from build123d import *

# Parameters (mm, degrees)
SKETCH1_W           = 150
SKETCH1_H           = 100
BOSS_EXTRUDE1_DEPTH = 3
SKETCH2_W           = 20
SKETCH2_H           = 3
CUT_EXTRUDE1_DEPTH  = 3
SKETCH3_W           = 3
SKETCH3_H           = 17
CUT_EXTRUDE2_DEPTH  = 3
SKETCH5_R           = 4.5
CUT_EXTRUDE4_DEPTH  = 30.5
SKETCH6_R           = 4.5
CUT_EXTRUDE5_DEPTH  = 10
SKETCH7_R           = 1
CUT_EXTRUDE6_DEPTH  = 10
SKETCH9_W           = 29.951530893
SKETCH9_H           = 14.675464834
CUT_EXTRUDE7_DEPTH  = 10
SKETCH10_W          = 6.632124697
SKETCH10_H          = 15.189704953
CUT_EXTRUDE8_DEPTH  = 10
CAVITY1_START       = -15
CAVITY1_OUTLINE_W   = 15
CAVITY1_OUTLINE_H   = 3
CAVITY1_DEPTH       = 3
CAVITY1_START_2     = 12
CAVITY1_2_OUTLINE_W = 15
CAVITY1_2_OUTLINE_H = 3
CAVITY1_2_DEPTH     = 3
SKETCH11_W          = 8.771519761
SKETCH11_H          = 15.403644459
CUT_EXTRUDE9_DEPTH  = 10


# Read off the part's stored shape, not the designer's step: Cavity1
with BuildPart() as part:
    # Sketch1 → Boss-Extrude1 (new body)
    with BuildSketch(Plane.XY):
        Rectangle(SKETCH1_W, SKETCH1_H)
    extrude(amount=BOSS_EXTRUDE1_DEPTH)

    # Sketch2 → Cut-Extrude1 (cut)
    with BuildSketch(Plane.XY.offset(3)):
        with Locations((65, 48.5)):
            Rectangle(SKETCH2_W, SKETCH2_H)
        with Locations((-65, 48.5)):
            Rectangle(SKETCH2_W, SKETCH2_H)
        with Locations((-65, -48.5)):
            Rectangle(SKETCH2_W, SKETCH2_H)
        with Locations((65, -48.5)):
            Rectangle(SKETCH2_W, SKETCH2_H)
    extrude(amount=-CUT_EXTRUDE1_DEPTH, mode=Mode.SUBTRACT)

    # Sketch3 → Cut-Extrude2 (cut)
    with BuildSketch(Plane.XY.offset(3)):
        with Locations((-73.5, 38.5)):
            Rectangle(SKETCH3_W, SKETCH3_H)
        with Locations((-73.5, -38.5)):
            Rectangle(SKETCH3_W, SKETCH3_H)
        with Locations((73.5, 38.5)):
            Rectangle(SKETCH3_W, SKETCH3_H)
        with Locations((73.5, -38.5)):
            Rectangle(SKETCH3_W, SKETCH3_H)
    extrude(amount=-CUT_EXTRUDE2_DEPTH, mode=Mode.SUBTRACT)

    # Sketch5 → Cut-Extrude4 (cut)
    with BuildSketch(Plane.XY.offset(3)):
        with Locations((50, 17.807715926)):
            Circle(SKETCH5_R)
        with Locations((-50, 17.807715926)):
            Circle(SKETCH5_R)
    extrude(amount=-CUT_EXTRUDE4_DEPTH, mode=Mode.SUBTRACT)

    # Sketch6 → Cut-Extrude5 (cut)
    with BuildSketch(Plane(origin=(0, 0, 0), x_dir=(-1, 0, 0), z_dir=(0, 0, -1))):
        with Locations((26.644067797, -29.026784983)):
            Circle(SKETCH6_R)
        with Locations((-26.644067797, -29.026784983)):
            Circle(SKETCH6_R)
    extrude(amount=-CUT_EXTRUDE5_DEPTH, mode=Mode.SUBTRACT)

    # Sketch7 → Cut-Extrude6 (cut)
    with BuildSketch(Plane.XY.offset(3)):
        with Locations((0, 18.473215017)):
            Circle(SKETCH7_R)
        with Locations((0, -29.026784983)):
            Circle(SKETCH7_R)
    extrude(amount=-CUT_EXTRUDE6_DEPTH, mode=Mode.SUBTRACT)

    # Sketch9 → Cut-Extrude7 (cut)
    with BuildSketch(Plane.XY.offset(3)):
        with Locations((52.201239556, -7.337732417)):
            Rectangle(SKETCH9_W, SKETCH9_H)
    extrude(amount=-CUT_EXTRUDE7_DEPTH, mode=Mode.SUBTRACT)

    # Sketch10 → Cut-Extrude8 (cut)
    with BuildSketch(Plane.XY.offset(3)):
        with Locations((0.32090926, -24.837591387)):
            Rectangle(SKETCH10_W, SKETCH10_H)
    extrude(amount=-CUT_EXTRUDE8_DEPTH, mode=Mode.SUBTRACT)

    # Cavity1 outline → Cavity1 (cut)
    with BuildSketch(Plane.YZ.offset(CAVITY1_START)):
        with Locations((-24.318956618, 1.5)):
            Rectangle(CAVITY1_OUTLINE_W, CAVITY1_OUTLINE_H)
    extrude(amount=CAVITY1_DEPTH, mode=Mode.SUBTRACT)

    # Cavity1 2 outline → Cavity1 2 (cut)
    with BuildSketch(Plane.YZ.offset(CAVITY1_START_2)):
        with Locations((-24.318956618, 1.5)):
            Rectangle(CAVITY1_2_OUTLINE_W, CAVITY1_2_OUTLINE_H)
    extrude(amount=CAVITY1_2_DEPTH, mode=Mode.SUBTRACT)

    # Sketch11 → Cut-Extrude9 (cut)
    with BuildSketch(Plane.XY.offset(3)):
        with Locations((0.32090926, 13.778489515)):
            Rectangle(SKETCH11_W, SKETCH11_H)
    extrude(amount=-CUT_EXTRUDE9_DEPTH, mode=Mode.SUBTRACT)


solid = part.part
Can you work these out from the model? Positions are in its coordinate system, mm. A direction names the side the tool comes from. Give positions to 0.01 mm unless a question says otherwise; leave off trailing zeros. Loops run counter-clockwise (first coordinate to the right, second up) from the corner with the lowest first, then second, coordinate; pieces in that order, holes last. Notation, with made-up numbers: (69, 79) - (92, 79) arc R15 ccw to (92, 104) - close; hole circle Ø8 at (59, 49.25). An arc over 180 degrees is marked (long way). Answer as a JSON object with one key per item and string values.
Q1. If we mould it in two halves opening along Y, with no side actions, what happens to faces 1 (the flat face through (52, 0, 2)), 2 (the flat face through (-1, 1, 3)), 3 (the flat face through (-74, -30, 2))? For each: pulls with the +Y half, pulls with the -Y half, needs draft (parallel to the pull), parting line crosses it, or undercut.
Geometry says:
{"face 1": "undercut", "face 2": "needs draft", "face 3": "pulls with the -Y half"}
Q2. Imagine slicing it at D-D on x = 50. Write out the boundary of the cut face in (y, z).
Geometry says:
{"outline": "(-50, 0) - (-14.68, 0) - (-14.68, 3) - (-50, 3) - close; (0, 0) - (13.31, 0) - (13.31, 3) - (0, 3) - close; (22.31, 0) - (50, 0) - (50, 3) - (22.31, 3) - close"}
Q3. Imagine slicing it at B-B on y = -22. Write out the boundary of the cut face in (x, z), plus the area to 3 significant figures.
Geometry says:
{"outline": "(-75, 0) - (-15, 0) - (-15, 3) - (-75, 3) - close; (-12, 0) - (-3, 0) - (-3, 3) - (-12, 3) - close; (3.64, 0) - (12, 0) - (12, 3) - (3.64, 3) - close; (15, 0) - (75, 0) - (75, 3) - (15, 3) - close", "area": "412 mm²"}
Q4. Imagine slicing it at A-A on x = -50. Write out the boundary of the cut face in (y, z), plus the area to 3 significant figures.
Geometry says:
{"outline": "(-50, 0) - (13.31, 0) - (13.31, 3) - (-50, 3) - close; (22.31, 0) - (50, 0) - (50, 3) - (22.31, 3) - close", "area": "273 mm²"}
Q5. Which directions (+Z, -Z, +X, -X, +Y, -Y) give clear straight access to the entire face, cutting with the end or side of a thin tool? Please do faces 4 (the flat face through (72, 38, 2)), 5 (the flat face through (72, -39, 2)), 6 (the flat face through (-1, 50, 1)), 7 (the flat face through (-72, 38, 2)), 8 (the flat face through (-4.065, 14, 2)).
Geometry says:
{"face 4": "+Z, -Z, +X, +Y", "face 5": "+Z, -Z, +X, -Y", "face 6": "+Z, -Z, +X, -X, +Y", "face 7": "+Z, -Z, -X, +Y", "face 8": "+Z, -Z"}
Q6. If I drill on L1, parallel to X at y = -29, z = 0.2; L2, parallel to Y at x = 50, z = 1.7; L3, parallel to Y at x = 47, z = 1.7, over which ranges is the centre line in solid material (lowest first)?
Geometry says:
{"L1": "-75 to -31.14, -22.14 to -15, -12 to -3, 3.64 to 12, 15 to 22.14, 31.14 to 75", "L2": "-50 to -14.68, 0 to 13.31, 22.31 to 50", "L3": "-50 to -14.68, 0 to 14.45, 21.16 to 50"}
Q7. Imagine slicing it at C-C on y = -7.5. Write out the boundary of the cut face in (x, z).
Geometry says:
{"outline": "(-75, 0) - (37.23, 0) - (37.23, 3) - (-75, 3) - close; (67.18, 0) - (75, 0) - (75, 3) - (67.18, 3) - close"}
Q8. Will these pins go through, and if not, where does the flat tip stop? P1, Ø1.5, axis at x = -62.5, z = 1.5, coming from the -Y side; P2, Ø1.5, axis at y = -35, z = 2, coming from the -X side.
Geometry says:
{"P1": "y = -47", "P2": "x = -72"}
